The listing builds one solid part. Answer for the finished solid, in the listing's coordinates (mm). A direction names the side the tool comes from. Give positions to 0.01 mm unless a question says otherwise; leave off trailing zeros. Order: outer loops, then holes, each group sorted by start corner. A loop starts at its lowest first (then second) coordinate and runs counter-clockwise, first axis right, second up. Notation, with made-up numbers: (21.25, -3.5) - (28.25, -3.5) arc R23 ccw to (28.25, 28.5) - close; hole circle Ø2 at (74, 7). An arc over 180 degrees is marked (long way). Write each question's results on one line, items separated by ' | '. Start each with the question number.
1. Flat-ended cylindrical pins translate along their axes: pin 1 (8 mm diameter, centred on x = 32.37, z = 32.37, fed in from -Y); pin 2 (6.5 mm diameter, centred on x = 32.37, z = -32.37, fed in from +Y); pin 3 (4 mm diameter, centred on x = -11.5, y = -10, fed in from -Z). Find the tip coordinate at first contact, or state that the pin passes through.
2. Which of the six approach directions +Z, -Z, +X, -X, +Y, -Y give full straight-line access (tool end or side, diameter ignored) to faces 1 (the face through (0, 0, 0)), 2 (the face through (-36, -4, 1))?
3. Find the intervals of material crossed by L1, parallel to Z at x = 1, y = -22.75; L2, parallel to Y at x = 20.5, z = -23, in increasing order.
4. Section B-B (x = 0) is taken. Give the vertices of the cut face in (y, z).
5. Determine the mould class of faces 3 (the face through (0, -2, 40)), 4 (the face through (-35.87, -1.97, -32.22)), 5 (the face through (0, -4, 0)), 6 (the face through (-28, -15, -21)) for opening direction Z: released by +Z, released by -Z, zero draft, split by the parting line, or undercut.
6. Section A-A (z = 0) is taken. Give the vertices of the cut face in (x, y).
7. Section C-C (y = -17.25) is taken. Give the vertices of the cut face in (x, z), and give its area (3 significant figures).
from build123d import *

# Parameters (mm, degrees)
F3_DEPTH = 4
F1_R     = 35
F1_R_2   = 33
F4_DEPTH = 26
F2_R     = 3.5
F5_DEPTH = 26.001
F6_R     = 33
F7_DEPTH = 22
F8_R     = 0.75


with BuildPart() as f3:
    # F0 (on Front) → F3 (new body)
    with BuildSketch(Plane.XZ):
        with BuildLine():
            Line((32.5, 40), (-32.5, 40))
            ThreePointArc((-32.5, 40), (-37.803301, 37.803301), (-40, 32.5))
            Line((-40, 32.5), (-40, -32.5))
            ThreePointArc((-40, -32.5), (-37.803301, -37.803301), (-32.5, -40))
            Line((-32.5, -40), (32.5, -40))
            ThreePointArc((32.5, -40), (37.803301, -37.803301), (40, -32.5))
            Line((40, -32.5), (40, 32.5))
            ThreePointArc((40, 32.5), (37.803301, 37.803301), (32.5, 40))
        make_face()
    extrude(amount=F3_DEPTH)

    # F1 (on face) → F4 (join)
    with BuildSketch(Plane.XZ):
        Circle(F1_R)
        Circle(F1_R_2, mode=Mode.SUBTRACT)
    extrude(amount=F4_DEPTH)

    # F2 (on face) → F5 (cut, through all)
    with BuildSketch(Plane.XZ):
        with Locations((-32.374369, 32.374369)):
            Circle(F2_R)
        with Locations((-32.374369, -32.374369)):
            Circle(F2_R)
        with Locations((32.374369, -32.374369)):
            Circle(F2_R)
        with Locations((32.374369, 32.374369)):
            Circle(F2_R)
    extrude(amount=F5_DEPTH, mode=Mode.SUBTRACT)

    # F6 (on face) → F7 (cut)
    with BuildSketch(Plane.XZ.offset(26)):
        Circle(F6_R)
    extrude(amount=-F7_DEPTH, mode=Mode.SUBTRACT)

    # F9: sweep along a path in F1
    with BuildLine(Plane.XZ) as f9_path:
        CenterArc((0, 0), 33, 0, 360)
    # F8 (on Right) → F9 (sweep, cut)
    with BuildSketch(Plane.YZ):
        with Locations((0, 34)):
            Circle(F8_R)
    sweep(path=f9_path.line, mode=Mode.SUBTRACT)


solid = f3.part
Reported:
1) pin 1: y = -4 | pin 2: through | pin 3: z = -33.69
2) face 1: +Z, -Z, +X, -X, +Y | face 2: -Y
3) L1: -34.99 to -32.98, 32.98 to 34.99 | L2: -4 to 0
4) outline: (-26, -35) - (-4, -35) - (-4, -40) - (0, -40) - (0, -34.75) arc R0.75 cw to (0, -33.25) - (0, 33.25) arc R0.75 cw to (0, 34.75) - (0, 40) - (-4, 40) - (-4, 35) - (-26, 35) - (-26, 33) - (-4, 33) - (-4, -33) - (-26, -33) - close
5) face 3: released by +Z | face 4: undercut | face 5: undercut | face 6: split by the parting line
6) outline: (-40, -4) - (-35, -4) - (-35, -26) - (-33, -26) - (-33, -4) - (33, -4) - (33, -26) - (35, -26) - (35, -4) - (40, -4) - (40, 0) - (34.75, 0) arc R0.75 cw to (33.25, 0) - (-33.25, 0) arc R0.75 cw to (-34.75, 0) - (-40, 0) - close
7) outline: circle Ø70 at (0, 0); hole circle Ø66 at (0, 0) | area: 427 mm²
